Read the model definition and answer for the solid it produces. Units are mm, in the model's axes. Round coordinates to 2 decimals unless told otherwise and drop trailing zeros. Loops run counter-clockwise (first coordinate to the right, second up) from the corner with the lowest first, then second, coordinate; pieces in that order, holes last. Notation, with made-up numbers: (56, -23) - (77, -23) arc R25 ccw to (77, 3) - close; hole circle Ø7 at (23, -27). An arc over 180 degrees is marked (long way). Use CSV: the item, a comma, the result in double quotes. Start each with the question number.
1. Find section C-C (y = 0.95). Give the vertices of the cut face in (x, z), and give its area (3 significant figures).
2. Consider line 1 along X through (y, z) = (0.8, 0); line 2 along Z through (x, y) = (3, 2); line 3 along X through (y, z) = (0.85, 25). Determine where each line is inside the solid, lowest interval first.
3. Find section D-D (x = 24.5). Give the vertices of the cut face in (y, z) (3 decimals).
4. Determine the mould class of faces 1 (the cylindrical face through (-0.77, 1.57, 3.47)), 2 (the flat face through (0, 3.175, -7)), 3 (the flat face through (0, 2, 28.5)) for opening direction Z: +Z half, -Z half, draft (parallel to the pull), parting line (faces both ways), or undercut.
5. Find section B-B (z = 0). Give the vertices of the cut face in (x, y) (3 decimals).
6. Find section A-A (x = 0). Give the vertices of the cut face in (y, z) (3 decimals), and give its area (3 significant figures).
from build123d import *

# Parameters (mm, degrees)
SKETCH1_R           = 3.556
SKETCH1_R_2         = 2.499995
BOSS_EXTRUDE1_DEPTH = 3.175


with BuildPart() as part:
    # Sketch1 → Boss-Extrude1 (new body)
    with BuildSketch(Plane(origin=(0, 0, 0), x_dir=(1, 0, 0), z_dir=(0, 1, 0))):
        with BuildLine():
            Line((-13.993314597, 28.4999938), (-25.9599938, 28.4999938))
            ThreePointArc((-25.9599938, 28.4999938), (-27.756045024, 27.756045024), (-28.4999938, 25.9599938))
            Line((-28.4999938, 25.9599938), (-28.4999938, 13.993314597))
            Line((-28.4999938, 13.993314597), (-28.4999938, -13.993314597))
            Line((-28.4999938, -13.993314597), (-28.4999938, -25.9599938))
            ThreePointArc((-28.4999938, -25.9599938), (-27.756045024, -27.756045024), (-25.9599938, -28.4999938))
            Line((-25.9599938, -28.4999938), (-13.993314597, -28.4999938))
            Line((-13.993314597, -28.4999938), (13.993314597, -28.4999938))
            Line((13.993314597, -28.4999938), (25.9599938, -28.4999938))
            ThreePointArc((25.9599938, -28.4999938), (27.756045024, -27.756045024), (28.4999938, -25.9599938))
            Line((28.4999938, -25.9599938), (28.4999938, -13.993314597))
            Line((28.4999938, -13.993314597), (28.4999938, 13.993314597))
            Line((28.4999938, 13.993314597), (28.4999938, 25.9599938))
            ThreePointArc((28.4999938, 25.9599938), (27.756045024, 27.756045024), (25.9599938, 28.4999938))
            Line((25.9599938, 28.4999938), (13.993314597, 28.4999938))
            Line((13.993314597, 28.4999938), (-13.993314597, 28.4999938))
        make_face()
        Circle(SKETCH1_R, mode=Mode.SUBTRACT)
        with Locations((-23.5000038, 23.5000038)):
            Circle(SKETCH1_R_2, mode=Mode.SUBTRACT)
        with Locations((23.5000038, 23.5000038)):
            Circle(SKETCH1_R_2, mode=Mode.SUBTRACT)
        with Locations((23.5000038, -23.5000038)):
            Circle(SKETCH1_R_2, mode=Mode.SUBTRACT)
        with Locations((-23.5000038, -23.5000038)):
            Circle(SKETCH1_R_2, mode=Mode.SUBTRACT)
    extrude(amount=BOSS_EXTRUDE1_DEPTH)


solid = part.part
Filled sheet:
1,outline,"(-28.5, -25.96) arc R2.54 ccw to (-25.96, -28.5) - (25.96, -28.5) arc R2.54 ccw to (28.5, -25.96) - (28.5, 25.96) arc R2.54 ccw to (25.96, 28.5) - (-25.96, 28.5) arc R2.54 ccw to (-28.5, 25.96) - close; hole circle Ø5 at (-23.5, -23.5); hole circle Ø5 at (-23.5, 23.5); hole circle Ø7.11 at (0, 0); hole circle Ø5 at (23.5, -23.5); hole circle Ø5 at (23.5, 23.5)"
1,area,"3,130 mm²"
2,line 1,"x = -28.5 to -3.56, 3.56 to 28.5"
2,line 2,"z = -28.5 to -1.91, 1.91 to 28.5"
2,line 3,"x = -28.5 to -25.5, -21.5 to 21.5, 25.5 to 28.5"
3,outline,"(0, -28.5) - (3.175, -28.5) - (3.175, -25.791) - (0, -25.791) - close; (0, -21.209) - (3.175, -21.209) - (3.175, 21.209) - (0, 21.209) - close; (0, 25.791) - (3.175, 25.791) - (3.175, 28.5) - (0, 28.5) - close"
4,face 1,"undercut"
4,face 2,"draft"
4,face 3,"+Z half"
5,outline,"(-28.5, 0) - (-3.556, 0) - (-3.556, 3.175) - (-28.5, 3.175) - close; (3.556, 0) - (28.5, 0) - (28.5, 3.175) - (3.556, 3.175) - close"
6,outline,"(0, -28.5) - (3.175, -28.5) - (3.175, -3.556) - (0, -3.556) - close; (0, 3.556) - (3.175, 3.556) - (3.175, 28.5) - (0, 28.5) - close"
6,area,"158 mm²"
